Input: part model. Units: mm. Frame: model coordinates. Round coordinates to 2 decimals unless told otherwise and drop trailing zeros. Order: outer loops, then holes, each group sorted by start corner. A loop starts at its lowest first (then second) coordinate and runs counter-clockwise, first axis right, second up. Notation, with made-up numbers: (5.5, -7) -> (27.5, -7) arc R24 ccw to (27.5, 29) -> close; hole circle Ø5 at (44.25, 81.5). An arc over 180 degrees is marked (long way). Answer as CSV lines item,"result". Start each with the question number.
1) Section query A-A, the plane z = 0. Output: boundary loops of the cut face in (x, y) (3 decimals), and give its area (3 significant figures).
2) Line query: L1, parallel to X at y = -0.5, z = -1; L2, parallel to Z at x = 4, y = -0.25; L3, parallel to Z at x = 24.5, y = 3.25. Output: solid intervals per line, ascending.
3) First-contact query: P1, Ø1, axis at y = -1, z = -1.5, coming from the -X side; P2, Ø1.5, axis at x = 11, y = 2.5, coming from the -Z side; P3, Ø4, axis at y = 0, z = 2.5, coming from the +X side. Flat tips, straight axial feed; report the tip coordinate or a pass-through.
4) Section query C-C, the plane x = 27. Output: boundary loops of the cut face in (y, z), and give its area (3 significant figures).
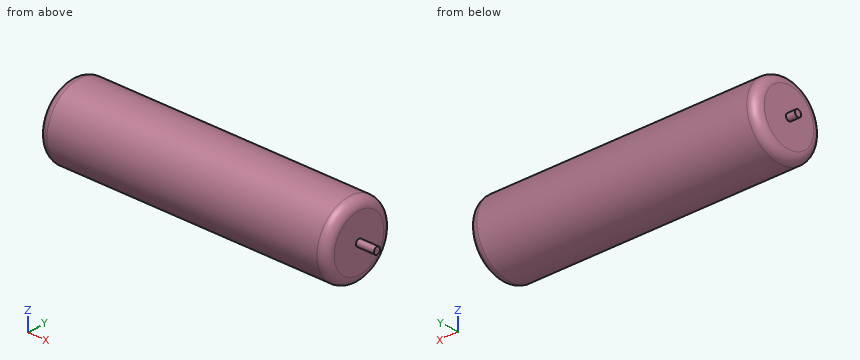
```python
from build123d import *

# Parameters (mm, degrees)
SKETCH_3_R           = 4
EXTRUDE_1_DEPTH      = 32
FILLET_1_R           = 1
EXTRUDE_2_DEPTH      = 1
EXTRUDE_2_DEPTH_BACK = 34
SKETCH_4_R           = 0.375


with BuildPart() as part:
    # 草图3 → 凸台-拉伸1 (new body)
    with BuildSketch(Plane(origin=(0, 0, 0), x_dir=(0, 0, -1), z_dir=(1, 0, 0))):
        Circle(SKETCH_3_R)
    extrude(amount=EXTRUDE_1_DEPTH)

    # 圆角1
    fillet_1_edges = [part.edges().sort_by_distance(p)[0] for p in [
        (0, 0, 4),
        (32, 0, 4),
    ]]
    fillet(fillet_1_edges, radius=FILLET_1_R)

    # 草图4 → 凸台-拉伸2 (add, two sides: drawn at the far end of the back side and taken through both)
    with BuildSketch(Plane.ZY.offset(-EXTRUDE_2_DEPTH_BACK)):
        Circle(SKETCH_4_R)
    extrude(amount=EXTRUDE_2_DEPTH + EXTRUDE_2_DEPTH_BACK)


solid = part.part
```
Findings:
1,outline,"(-1, -0.375) -> (0, -0.375) -> (0, -3) arc R1 ccw to (1, -4) -> (31, -4) arc R1 ccw to (32, -3) -> (32, -0.375) -> (34, -0.375) -> (34, 0.375) -> (32, 0.375) -> (32, 3) arc R1 ccw to (31, 4) -> (1, 4) arc R1 ccw to (0, 3) -> (0, 0.375) -> (-1, 0.375) -> close"
1,area,"257 mm^2"
2,L1,"x = 0 to 32"
2,L2,"z = -3.99 to 3.99"
2,L3,"z = -2.33 to 2.33"
3,P1,"stops at x = 0"
3,P2,"stops at z = -3.6"
3,P3,"stops at x = 32"
4,outline,"circle Ø8 at (0, 0)"
4,area,"50.3 mm^2"
